Source: CAD feature listing. Evaluate the final solid. Frame: model axes, mm. A direction names the side the tool comes from. Give positions to 0.01 mm unless a question says otherwise; leave off trailing zeros. Loops run counter-clockwise (first coordinate to the right, second up) from the corner with the lowest first, then second, coordinate; pieces in that order, holes last. Notation, with made-up numbers: (86.25, 14.25) -> (112.25, 14.25) arc R26 ccw to (112.25, 38.25) -> close; hole circle Ø7 at (49, 73). An arc over 180 degrees is marked (long way). Put each result on its own line as item: value.
```python
from build123d import *

# Parameters (mm, degrees)
PROFILEBOSS_EXTRUDE3_DEPTH            = 41.74
SKETCH5_R                             = 1.55
SHROUDHOLESCUT_EXTRUDE1_DEPTH         = 66.944883046
SIDECUTOUTCUT_EXTRUDE3_DEPTH          = 66.944883046
FRONTCUTOUTCUT_EXTRUDE4_DEPTH         = 65.457176482
SKETCH11_R                            = 2.25
DRAGCHAINMOUNTHOLESCUT_EXTRUDE6_DEPTH = 3.1
CUT_EXTRUDE7_DEPTH                    = 2


with BuildPart() as part:
    # Sketch4 → ProfileBoss-Extrude3 (new body)
    with BuildSketch(Plane(origin=(0, 0, 0), x_dir=(1, 0, 0), z_dir=(0, 1, 0))):
        Polygon((0, 0), (0, 8.4), (45.5, 8.4), (45.5, 0), (47.5, 0), (47.5, 12.5), (-2, 12.5), (-2, 0), align=None)
    extrude(amount=PROFILEBOSS_EXTRUDE3_DEPTH)

    # Sketch5 → ShroudHolesCut-Extrude1 (cut, through all)
    with BuildSketch(Plane(origin=(47.5, 0, 0), x_dir=(0, 0, -1), z_dir=(1, 0, 0))):
        with Locations((3.1, 3.1)):
            Circle(SKETCH5_R)
    extrude(amount=-SHROUDHOLESCUT_EXTRUDE1_DEPTH, mode=Mode.SUBTRACT)

    # SideCutoutSketch9 → SideCutoutCut-Extrude3 (cut, through all)
    with BuildSketch(Plane.ZY.offset(2)):
        Polygon((0, 41.74), (-8.4, 41.74), (-8.4, 27.59), (0, 13.74), align=None)
    extrude(amount=-SIDECUTOUTCUT_EXTRUDE3_DEPTH, mode=Mode.SUBTRACT)

    # FrontCutoutSketch7 → FrontCutoutCut-Extrude4 (cut, through all)
    with BuildSketch(Plane(origin=(0, 0, -12.5), x_dir=(-1, 0, 0), z_dir=(0, 0, -1))):
        Polygon((-21, 41.74), (-21, 27.59), (-34.85, 13.74), (-47.5, 13.74), (-47.5, 41.74), align=None)
    extrude(amount=-FRONTCUTOUTCUT_EXTRUDE4_DEPTH, mode=Mode.SUBTRACT)

    # Sketch11 → DragChainMountHolesCut-Extrude6 (cut)
    with BuildSketch(Plane(origin=(0, 0, -12.5), x_dir=(-1, 0, 0), z_dir=(0, 0, -1))):
        with Locations((-3, 21.74)):
            Circle(SKETCH11_R)
        with Locations((-10.5, 27.74)):
            Circle(SKETCH11_R)
        with Locations((-3, 33.74)):
            Circle(SKETCH11_R)
    extrude(amount=-DRAGCHAINMOUNTHOLESCUT_EXTRUDE6_DEPTH, mode=Mode.SUBTRACT)

    # Sketch13 → Cut-Extrude7 (cut)
    with BuildSketch(Plane.XY.offset(-8.4)):
        Polygon((21.142710497, 27.447289503), (34.85, 13.74), (45.5, 13.74), (45.5, 0), (0, 0), (0, 13.74), (21.142710497, 13.74), align=None)
    extrude(amount=-CUT_EXTRUDE7_DEPTH, mode=Mode.SUBTRACT)


solid = part.part
```
(1) Section D-D on y = 6. Return loops of the section in (x, z).
Calculated:
outline: (-2, -12.5) -> (47.5, -12.5) -> (47.5, 0) -> (45.5, 0) -> (45.5, -10.4) -> (0, -10.4) -> (0, 0) -> (-2, 0) -> close
(2) Draft query along X for faces 5 (the flat face through (9, 41.74, -10)), 6 (the cylindrical face through (10.988, 25.544, -10.972)), 7 (the flat face through (21, 35, -10)). Return one class per face: released by +X, released by -X, zero draft, split by the parting line, or undercut.
Calculated:
face 5: zero draft
face 6: undercut
face 7: released by +X
(3) First-contact query: P1, Ø2, axis at y = 33, z = -11, coming from the +X side; P2, Ø3.5, axis at x = 3, y = 33.74, coming from the -Z side; P3, Ø7, axis at x = 12.5, y = 27.5, coming from the +Z side; P4, Ø12, axis at x = 25.5, y = 26, coming from the -Z side. Flat tips, straight axial feed; report the tip coordinate or a pass-through.
Calculated:
P1: stops at x = 21
P2: stops at z = -9.4
P3: stops at z = -8.4
P4: stops at z = -12.5
(4) Section A-A on x = 3. Return loops of the section in (y, z), then the cut area to 3 significant figures.
Calculated:
outline: (0, -12.5) -> (19.49, -12.5) -> (19.49, -9.4) -> (23.99, -9.4) -> (23.99, -12.5) -> (31.49, -12.5) -> (31.49, -9.4) -> (35.99, -9.4) -> (35.99, -12.5) -> (41.74, -12.5) -> (41.74, -8.4) -> (13.74, -8.4) -> (13.74, -10.4) -> (0, -10.4) -> close
area: 116 mm²
(5) Line query: probe 1 along Y at (x, z) = (3, -10.65); probe 2 along X at (y, z) = (10, -10); probe 3 along Y at (x, z) = (10.5, -11.35). Output: solid intervals per line, ascending. Write a range as from..to.
Calculated:
probe 1: y = 0..19.49, 23.99..31.49, 35.99..41.74
probe 2: x = -2..0, 45.5..47.5
probe 3: y = 0..25.49, 29.99..41.74
(6) Reachability of faces 1 (the cylindrical face through (3.488, 19.544, -10.972)), 2 (the cylindrical face through (-0.986, 3.566, -4.578)), 3 (the flat face through (21.143, 20, -9)), 4 (the flat face through (0, 11, -5)) from +Z, -Z, +X, -X, +Y, -Y: full face, straight path, thin tool, end or side. Return the list, or none.
Calculated:
face 1: -Z
face 2: +X, -X
face 3: +Z, +X, +Y, -Y
face 4: +Z, -Y
(7) Section B-B on z = -3.75. Return loops of the section in (x, y).
Calculated:
outline: (-2, 0) -> (0, 0) -> (0, 1.69) -> (-2, 1.69) -> close; (-2, 4.51) -> (0, 4.51) -> (0, 19.92) -> (-2, 19.92) -> close; (45.5, 0) -> (47.5, 0) -> (47.5, 1.69) -> (45.5, 1.69) -> close; (45.5, 4.51) -> (47.5, 4.51) -> (47.5, 13.74) -> (45.5, 13.74) -> close
(8) Section C-C on y = 33.74. Return loops of the section in (x, z).
Calculated:
outline: (-2, -12.5) -> (0.75, -12.5) -> (0.75, -9.4) -> (5.25, -9.4) -> (5.25, -12.5) -> (21, -12.5) -> (21, -8.4) -> (-2, -8.4) -> close
